Design review of the part built by this model. Coordinates are the model's own, in mm. Coordinates: 2 decimals unless noted, no trailing zeros. Loops run counter-clockwise (first coordinate to the right, second up) from the corner with the lowest first, then second, coordinate; pieces in that order, holes last. Notation, with made-up numbers: (26.25, 53) - (62.25, 53) arc R20 cw to (62.25, 62) - close; hole circle Ø8 at (-31.75, 27). An arc over 180 degrees is marked (long way). Use one line per item in the form item = value. Start each with the question number.
(1) Add section B-B (z = 4.5). State the section outline as (x, y) points, plus the area to 3 significant figures.
(2) Add section A-A (x = 13). State the section outline as (y, z) points, plus the area to 3 significant figures.
(3) For L1, parallel to Y at x = 31, z = 2.25; L2, parallel to Z at x = 63.5, y = 22.5; L3, parallel to Y at x = 5, z = 2, list the stretches that pass through material, from the lowest coordinate up.
(4) Clearance check with a flat-ended pin moving along its axis: pin 1 Ø1.5 at (x, z) = (26, 4) entering from +Y. State where the tip first meets the part, or that it passes through.
```python
from build123d import *

# Parameters (mm, degrees)
SKETCH1_W           = 82.55
SKETCH1_H           = 25.4
BOSS_EXTRUDE1_DEPTH = 6.35
CHAMFER1_SIZE       = 5.08
CHAMFER1_SIZE2      = 8.798818102


with BuildPart() as part:
    # Sketch1 → Boss-Extrude1 (new body)
    with BuildSketch(Plane.XY):
        with Locations((41.275, 12.7)):
            Rectangle(SKETCH1_W, SKETCH1_H)
    extrude(amount=BOSS_EXTRUDE1_DEPTH)

    # Chamfer1
    chamfer1_edges = [part.edges().sort_by_distance(p)[0] for p in [
        (41.275, 25.4, 6.35),
    ]]
    chamfer1_side = [part.faces().sort_by_distance(p)[0] for p in [
        (41.275, 25.4, 3.175),
    ]]
    chamfer(chamfer1_edges, length=CHAMFER1_SIZE, length2=CHAMFER1_SIZE2, reference=chamfer1_side[0])


solid = part.part
```
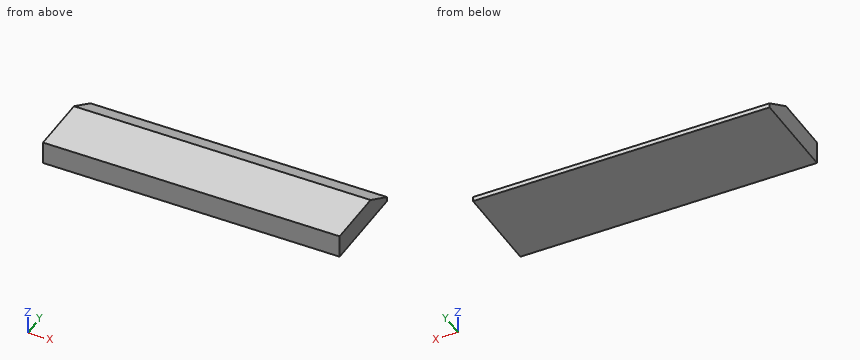
Computed values:
q1.outline = (0, 0) - (82.55, 0) - (82.55, 19.81) - (0, 19.81) - close
q1.area = 1,630 mm^2
q2.outline = (0, 0) - (25.4, 0) - (25.4, 1.27) - (16.6, 6.35) - (0, 6.35) - close
q2.area = 139 mm^2
q3.L1 = 0 to 23.7
q3.L2 = 0 to 2.94
q3.L3 = 0 to 24.14
q4.pin_1 = 21.97
